Source: CAD feature listing. Evaluate the final solid. Frame: model axes, mm. A direction names the side the tool comes from. Coordinates: 2 decimals unless noted, no trailing zeros. Loops run counter-clockwise (first coordinate to the right, second up) from the corner with the lowest first, then second, coordinate; pieces in that order, holes last.
from build123d import *

# Parameters (mm, degrees)
BOSS_EXTRUDE2_DEPTH = 50
CUT_EXTRUDE1_DEPTH  = 50
FILLET1_R           = 5
SKETCH10_W          = 50
SKETCH10_H          = 5.46
BOSS_EXTRUDE4_DEPTH = 10
SKETCH5_W           = 50
SKETCH5_H           = 5.464
BOSS_EXTRUDE5_DEPTH = 10
SKETCH11_R          = 1.5
CUT_EXTRUDE2_DEPTH  = 10
SKETCH12_R          = 1.5
CUT_EXTRUDE3_DEPTH  = 10
FILLET2_R           = 5
FILLET3_R           = 5
CUT_EXTRUDE8_DEPTH  = 8.5
SKETCH18_W          = 15.2
SKETCH18_H          = 46.4
CUT_EXTRUDE14_DEPTH = 1.8
SKETCH19_W          = 15.2
SKETCH19_H          = 46.4
CUT_EXTRUDE15_DEPTH = 1.8
SKETCH16_W          = 40
SKETCH16_H          = 2
CUT_EXTRUDE16_DEPTH = 10
SKETCH17_W          = 40
SKETCH17_H          = 2
CUT_EXTRUDE17_DEPTH = 10
SKETCH13_R          = 1.6
CUT_EXTRUDE18_DEPTH = 10
SKETCH20_R          = 2.5
CUT_EXTRUDE19_DEPTH = 1.5


with BuildPart() as part:
    # Sketch1 → Boss-Extrude2 (new body)
    with BuildSketch(Plane.XY):
        Polygon((-87.5, 0), (87.5, 0), (50.05, 85), (-50.05, 85), align=None)
    extrude(amount=BOSS_EXTRUDE2_DEPTH)

    # Sketch3 → Cut-Extrude1 (cut)
    with BuildSketch(Plane.XY.offset(50)):
        Polygon((-81.5, 0), (81.5, 0), (45.05, 80), (-45.05, 80), align=None)
    extrude(amount=-CUT_EXTRUDE1_DEPTH, mode=Mode.SUBTRACT)

    # Fillet1
    fillet1_edges = [part.edges().sort_by_distance(p)[0] for p in [
        (-45.05, 80, 25),
        (45.05, 80, 25),
    ]]
    fillet(fillet1_edges, radius=FILLET1_R)

    # Sketch10 → Boss-Extrude4 (add, along a direction that is not the sketch's normal)
    with BuildSketch(Plane(origin=(-73.275840836, 32.284473404, 0), x_dir=(0, 0, 1), z_dir=(-0.915116485, 0.403189557, 0))):
        with Locations((25, -32.549086253)):
            Rectangle(SKETCH10_W, SKETCH10_H)
    extrude(amount=BOSS_EXTRUDE4_DEPTH, dir=(-1, 0, 0))

    # Sketch5 → Boss-Extrude5 (add, along a direction that is not the sketch's normal)
    with BuildSketch(Plane(origin=(73.275840836, 32.284473404, 0), x_dir=(0, 0, -1), z_dir=(0.915116485, 0.403189557, 0))):
        with Locations((-25, -32.547086253)):
            Rectangle(SKETCH5_W, SKETCH5_H)
    extrude(amount=BOSS_EXTRUDE5_DEPTH, dir=(1, 0, 0))

    # Sketch11 → Cut-Extrude2 (cut)
    with BuildSketch(Plane(origin=(0, 4.996536008, 0), x_dir=(1, 0, 0), z_dir=(0, 1, 0))):
        with Locations((-92.5, -14)):
            Circle(SKETCH11_R)
        with Locations((-92.5, -36)):
            Circle(SKETCH11_R)
    extrude(amount=-CUT_EXTRUDE2_DEPTH, mode=Mode.SUBTRACT)

    # Sketch12 → Cut-Extrude3 (cut)
    with BuildSketch(Plane(origin=(0, 5.000196474, 0), x_dir=(1, 0, 0), z_dir=(0, 1, 0))):
        with Locations((92.5, -14)):
            Circle(SKETCH12_R)
        with Locations((92.5, -36)):
            Circle(SKETCH12_R)
    extrude(amount=-CUT_EXTRUDE3_DEPTH, mode=Mode.SUBTRACT)

    # Fillet2
    fillet2_edges = [part.edges().sort_by_distance(p)[0] for p in [
        (-85.298585018, 4.996536008, 25),
        (85.29697226, 5.000196474, 25),
    ]]
    fillet(fillet2_edges, radius=FILLET2_R)

    # Fillet3
    fillet3_edges = [part.edges().sort_by_distance(p)[0] for p in [
        (-50.05, 85, 25),
        (50.05, 85, 25),
    ]]
    fillet(fillet3_edges, radius=FILLET3_R)

    # Sketch15 → Cut-Extrude8 (cut)
    with BuildSketch(Plane(origin=(0, 85, 0), x_dir=(1, 0, 0), z_dir=(0, 1, 0))):
        with BuildLine():
            Line((-23.999155874, -20.87), (-23.999155874, -29.13))
            ThreePointArc((-23.999155874, -29.13), (-27.999155874, -33.13), (-31.999155874, -29.13))
            Line((-31.999155874, -29.13), (-31.999155874, -20.87))
            ThreePointArc((-31.999155874, -20.87), (-27.999155874, -16.87), (-23.999155874, -20.87))
        make_face()
        with BuildLine():
            Line((32.000844126, -20.87), (32.000844126, -29.13))
            ThreePointArc((32.000844126, -29.13), (28.000844126, -33.13), (24.000844126, -29.13))
            Line((24.000844126, -29.13), (24.000844126, -20.87))
            ThreePointArc((24.000844126, -20.87), (28.000844126, -16.87), (32.000844126, -20.87))
        make_face()
    extrude(amount=-CUT_EXTRUDE8_DEPTH, mode=Mode.SUBTRACT)

    # Sketch18 → Cut-Extrude14 (cut)
    with BuildSketch(Plane.XZ):
        with Locations((88.1, 25)):
            Rectangle(SKETCH18_W, SKETCH18_H)
    extrude(amount=-CUT_EXTRUDE14_DEPTH, mode=Mode.SUBTRACT)

    # Sketch19 → Cut-Extrude15 (cut)
    with BuildSketch(Plane.XZ):
        with Locations((-88.1, 25)):
            Rectangle(SKETCH19_W, SKETCH19_H)
    extrude(amount=-CUT_EXTRUDE15_DEPTH, mode=Mode.SUBTRACT)

    # Sketch16 → Cut-Extrude16 (cut)
    with BuildSketch(Plane(origin=(73.275840836, 32.284473404, 0), x_dir=(0, 0, -1), z_dir=(0.915116485, 0.403189557, 0))):
        with Locations((-25, 48.344419756)):
            Rectangle(SKETCH16_W, SKETCH16_H)
        with Locations((-25, -22.554242128)):
            Rectangle(SKETCH16_W, SKETCH16_H)
    extrude(amount=-CUT_EXTRUDE16_DEPTH, mode=Mode.SUBTRACT)

    # Sketch17 → Cut-Extrude17 (cut)
    with BuildSketch(Plane(origin=(-73.275840836, 32.284473404, 0), x_dir=(0, 0, 1), z_dir=(-0.915116485, 0.403189557, 0))):
        with Locations((25, 48.344419756)):
            Rectangle(SKETCH17_W, SKETCH17_H)
        with Locations((25, -22.558242128)):
            Rectangle(SKETCH17_W, SKETCH17_H)
    extrude(amount=-CUT_EXTRUDE17_DEPTH, mode=Mode.SUBTRACT)

    # Sketch13 → Cut-Extrude18 (cut)
    with BuildSketch(Plane(origin=(0, 85, 0), x_dir=(1, 0, 0), z_dir=(0, 1, 0))):
        with Locations((0.000844126, -10.945)):
            Circle(SKETCH13_R)
        with Locations((-8.129155874, -39.055)):
            Circle(SKETCH13_R)
        with Locations((8.130844126, -39.055)):
            Circle(SKETCH13_R)
    extrude(amount=-CUT_EXTRUDE18_DEPTH, mode=Mode.SUBTRACT)

    # Sketch20 → Cut-Extrude19 (cut)
    with BuildSketch(Plane.XZ.offset(-80)):
        with Locations((-8.129155874, 39.055)):
            Circle(SKETCH20_R)
        with Locations((8.130844126, 39.055)):
            Circle(SKETCH20_R)
        with Locations((0.000844126, 10.945)):
            Circle(SKETCH20_R)
    extrude(amount=-CUT_EXTRUDE19_DEPTH, mode=Mode.SUBTRACT)


solid = part.part
Q1. Draft query along Z for faces 1 (the cylindrical face through (-44.572, 79.183, 24.65)), 2 (the flat face through (50.439, 76.144, 25.28)). Return one class per face: +Z half, -Z half, draft (parallel to the pull), parting line (faces both ways), or undercut.
Q2. Section A-A, the plane y = 44. Return the cut outline in (x, z).
Q3. Section B-B, the plane y = 31.5. Return the cut outline in (x, z), plus the area to 3 significant figures.
Q4. Access query for faces 3 (the flat face through (-80, 11, 5)), 4 (the cylindrical face through (44.572, 79.183, 24.65)), 5 (the cylindrical face through (10.44, 80.74, 38.1)). Directions: +Z, -Z, +X, -X, +Y, -Y. A direction counts if a zero-diameter tool reaches every point of the face in a straight line with its end or side. Return the directions, or none.
Q5. Contact query for flat-ended pins moving along their axis: pin 1 Ø8 at (y, z) = (22.5, 6.5) entering from -X; pin 2 Ø0.5 at (y, z) = (0.5, 18.5) entering from +X; pin 3 Ø3 at (y, z) = (31.5, 20) entering from +X. Output: stop coordinate, or through.
Q6. Line query: line 1 along Z through (x, y) = (92.5, 4.05); line 2 along X through (y, z) = (2, 36); line 3 along Y through (x, z) = (41, 8). Output: solid intervals per line, ascending.
Q7. Section C-C, the plane x = -17. Return the cut outline in (y, z).
Derived:
1. face 1: draft
1. face 2: undercut
2. outline: (-68.11, 0) - (-61.45, 0) - (-61.45, 50) - (-68.11, 50) - close; (61.45, 0) - (68.11, 0) - (68.11, 50) - (61.45, 50) - close
3. outline: (-73.62, 0) - (-67.15, 0) - (-67.15, 50) - (-73.62, 50) - close; (67.15, 0) - (73.62, 0) - (73.62, 50) - (67.15, 50) - close
3. area: 647 mm2
4. face 3: none
4. face 4: +Z, -Z, -Y
4. face 5: -Y
5. pin 1: stops at x = -79.35
5. pin 2: stops at x = 97.39
5. pin 3: stops at x = 74.28
6. line 1: z = 0 to 12.5, 15.5 to 34.5, 37.5 to 50
6. line 2: x = -96.62 to -94, -91 to -80.59, 80.59 to 91, 94 to 96.62
6. line 3: y = 80 to 85
7. outline: (80, 0) - (85, 0) - (85, 50) - (80, 50) - close
